from build123d import *

# Parameters (mm, degrees)
F0_R     = 38.1
F0_R_2   = 2.15265
F1_DEPTH = 3.175


with BuildPart() as f1:
    # F0 (on Top) → F1 (new body)
    with BuildSketch(Plane.XY):
        Circle(F0_R)
        with Locations((-9.525, -16.497784)):
            Circle(F0_R_2, mode=Mode.SUBTRACT)
        with Locations((9.525, -16.497784)):
            Circle(F0_R_2, mode=Mode.SUBTRACT)
        with Locations((-19.05, 0)):
            Circle(F0_R_2, mode=Mode.SUBTRACT)
        with Locations((-9.525, 16.497784)):
            Circle(F0_R_2, mode=Mode.SUBTRACT)
        Polygon((7.405672, 0), (3.702836, -6.4135), (-3.702836, -6.4135), (-7.405672, 0), (-3.702836, 6.4135), (3.702836, 6.4135), align=None, mode=Mode.SUBTRACT)
        with Locations((9.525, 16.497784)):
            Circle(F0_R_2, mode=Mode.SUBTRACT)
        with Locations((19.05, 0)):
            Circle(F0_R_2, mode=Mode.SUBTRACT)
    extrude(amount=F1_DEPTH)


solid = f1.part
Check sheet for the modelled part. Datum: model origin and axes. Units: mm. A direction names the side the tool comes from. Round coordinates to 2 decimals unless told otherwise and drop trailing zeros. Loops run counter-clockwise (first coordinate to the right, second up) from the corner with the lowest first, then second, coordinate; pieces in that order, holes last.
1. Sectioned sample at A-A on y = -4. Record the boundary of the cut face in (x, z) (3 decimals).
2. Set-up check for faces 1 (the flat face through (8, 1, 0)), 2 (the flat face through (0, -6.414, 2)): record each of +Z, -Z, +X, -X, +Y, -Y from which the full face is reachable in a straight line by a thin tool's end or side.
3. Sectioned sample at C-C on z = 0.6. Give the number of separate pieces and of enclosed holes in the cut face, and give its area (3 significant figures).
4. Sectioned sample at B-B on x = -5. Record the boundary of the cut face in (y, z) (1 decimal).
5. Scan lines: probe 1 along Y at (x, z) = (4.5, 0.4); probe 2 along Y at (x, z) = (-5, 0.5); probe 3 along X at (y, z) = (16, 2.4). Record each from-to range of solid material in increasing order.
6. Gauge pin test, flat ends, axial feed: pin 1 Ø2.5 at (x, y) = (9.52, -16.5) entering from -Z; pin 2 Ø1.5 at (y, z) = (-8, 2.5) entering from +X; pin 3 Ø1 at (x, z) = (-0.5, 1.5) entering from +Y. Record the tip position at first contact, or that the pin passes through.
7. Sectioned sample at D-D on x = 9.5. Record the boundary of the cut face in (y, z) (3 decimals).
8. Mould release check, pull along Y, two halves, no side actions. Record for faces 3 (the cylindrical face through (-7.536, -17.322, 1.565)), 4 (the cylindrical face through (-30.235, -23.183, 1.565)), 5 (the cylindrical face through (21.103, 0.647, 1.565)), 6 (the flat face through (8, 1, 3.175)): released by +Y, released by -Y, zero draft, split by the parting line, or undercut.
Recorded:
1. outline: (-37.889, 0) - (-5.096, 0) - (-5.096, 3.175) - (-37.889, 3.175) - close; (5.096, 0) - (37.889, 0) - (37.889, 3.175) - (5.096, 3.175) - close
2. face 1: -Z, +X, -X, +Y, -Y
2. face 2: +Z, -Z
3. separate pieces: 1
3. enclosed holes: 7
3. area: 4,330 mm2
4. outline: (-37.8, 0) - (-4.2, 0) - (-4.2, 3.2) - (-37.8, 3.2) - close; (4.2, 0) - (37.8, 0) - (37.8, 3.2) - (4.2, 3.2) - close
5. probe 1: y = -37.83 to -5.03, 5.03 to 37.83
5. probe 2: y = -37.77 to -4.17, 4.17 to 37.77
5. probe 3: x = -34.58 to -11.62, -7.43 to 7.43, 11.62 to 34.58
6. pin 1: passes through
6. pin 2: stops at x = 37.4
6. pin 3: stops at y = 38.1
7. outline: (-36.897, 0) - (-18.65, 0) - (-18.65, 3.175) - (-36.897, 3.175) - close; (-14.345, 0) - (14.345, 0) - (14.345, 3.175) - (-14.345, 3.175) - close; (18.65, 0) - (36.897, 0) - (36.897, 3.175) - (18.65, 3.175) - close
8. face 3: undercut
8. face 4: split by the parting line
8. face 5: undercut
8. face 6: zero draft
